Here's the drawing with two shaded views (mm, measured from the low corner). I have some questions. Coordinates: 2 decimals unless noted, no trailing zeros. Write each loop counter-clockwise with the first axis right and the second up, starting at its lowest first coordinate (ties: lowest second). Pieces come first, ordered by that corner, then holes. Notation, with made-up numbers: (-5.5, 83.5) -> (30.5, 83.5) arc R20 ccw to (30.5, 112.5) -> close; hole circle Ø3 at (72.25, 7). An arc over 180 degrees is marked (long way). Put each result on its own line as item: value. Start each with the question number.
Item 1: I need wall thicknesses on line 1 (X direction, y = 75, z = 1.5); line 2 (X direction, y = 149, z = 9.75); line 3 (Y direction, x = 39, z = 1.5). Which ranges of each line are inside material? Lowest first, please. Write a range as [from, to].
Item 2: I want a section at C-C, the plane z = 21.5. List the corners of the cut face in (x, y) for me (1 decimal).
Item 3: For pin 1 (12 mm diameter, centred on y = 125, z = 23.5, fed in from +X); pin 2 (1.2 mm diameter, centred on x = 28.5, z = 2.5, fed in from -Y); pin 3 (1.2 mm diameter, centred on x = 41, z = 3, fed in from +Y); pin 4 (10 mm diameter, centred on x = 19, z = 15.5, fed in from +Y), each with a flat end and sliding along its axis, tell me the tip position at first contact or that it passes through.
Item 4: I want a section at D-D, the plane y = 126.5. List the corners of the cut face in (x, z) for me, then the cut area to 3 significant figures.
Item 5: I want a section at A-A, the plane y = 107. List the corners of the cut face in (x, z) for me, then the cut area to 3 significant figures.
Item 6: I want a section at B-B, the plane x = 50. List the corners of the cut face in (y, z) for me.
Item 7: If we mould it in two halves opening along Y, with no side actions, what happens to the marked faces 1, 2 and 3? For each: released by +Y, released by -Y, zero draft, split by the parting line, or undercut.
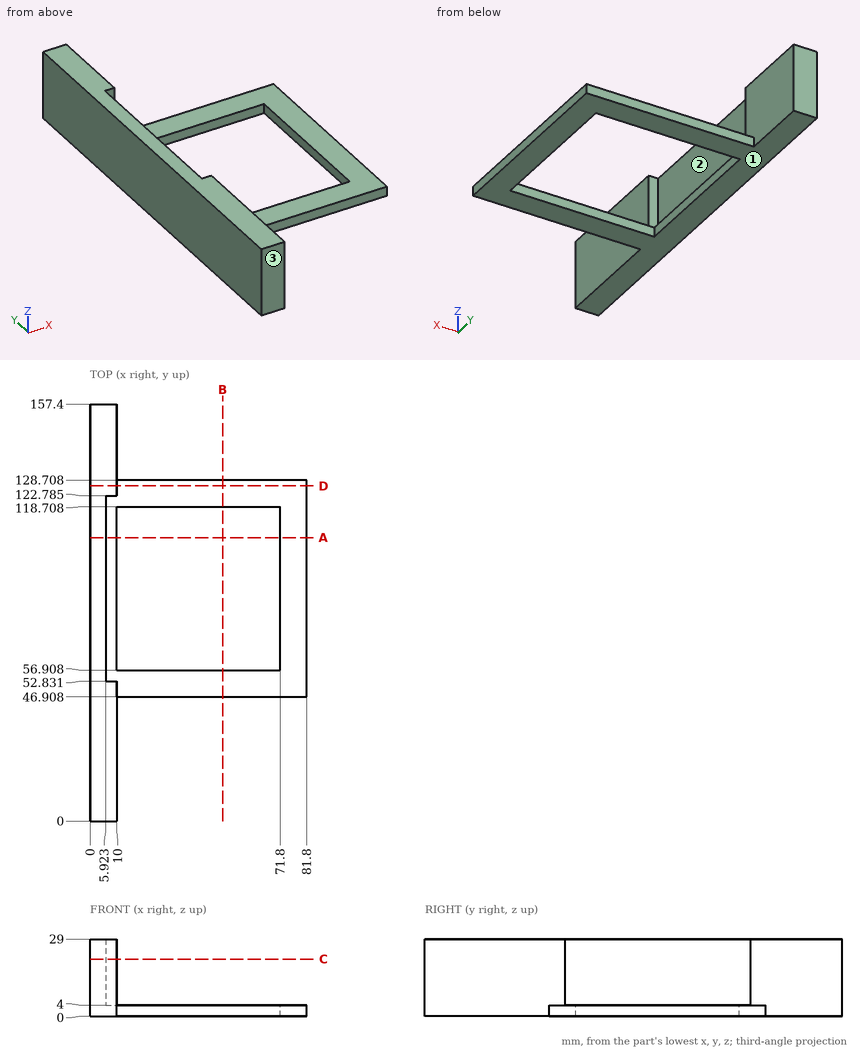
Calculated:
1. line 1: x = [0, 10], [71.8, 81.8]
1. line 2: x = [0, 10]
1. line 3: y = [46.91, 56.91], [118.71, 128.71]
2. outline: (0, 0) -> (10, 0) -> (10, 52.8) -> (5.9, 52.8) -> (5.9, 122.8) -> (10, 122.8) -> (10, 157.4) -> (0, 157.4) -> close
3. pin 1: stops at x = 10
3. pin 2: stops at y = 46.91
3. pin 3: stops at y = 128.71
3. pin 4: passes through
4. outline: (0, 0) -> (81.8, 0) -> (81.8, 4) -> (10, 4) -> (10, 29) -> (0, 29) -> close
4. area: 577 mm2
5. outline: (0, 0) -> (10, 0) -> (10, 4) -> (5.92, 4) -> (5.92, 29) -> (0, 29) -> close; (71.8, 0) -> (81.8, 0) -> (81.8, 4) -> (71.8, 4) -> close
5. area: 228 mm2
6. outline: (46.91, 0) -> (56.91, 0) -> (56.91, 4) -> (46.91, 4) -> close; (118.71, 0) -> (128.71, 0) -> (128.71, 4) -> (118.71, 4) -> close
7. face 1: zero draft
7. face 2: undercut
7. face 3: released by -Y
